Source: CAD feature listing. Evaluate the final solid. Frame: model axes, mm. A direction names the side the tool comes from. Round coordinates to 2 decimals unless told otherwise and drop trailing zeros. Loops run counter-clockwise (first coordinate to the right, second up) from the corner with the lowest first, then second, coordinate; pieces in that order, holes last. Notation, with made-up numbers: (51, 22) - (72, 22) arc R17 ccw to (72, 27) - close; hole circle Ø5 at (16.25, 52.25). An arc over 180 degrees is marked (long way). One line per question, with ' | ' between items. Start each with the question number.
1. Access query for faces 4 (the flat face through (20, 35, 1)), 5 (the flat face through (20, 59, 14)), 6 (the flat face through (20, 54, 19)). Directions: +Z, -Z, +X, -X, +Y, -Y. A direction counts if a zero-diameter tool reaches every point of the face in a straight line with its end or side. Return the directions, or none.
2. Cut plane B-B (x = 20). Return loops of the section in (y, z).
3. Mould query, pull axis Z, two halves, no side actions, for faces 1 (the flat face through (20, 5, -20)), 2 (the cylindrical face through (37.038, 56.535, 18.996)), 3 (the flat face through (20, 27, 6)). Classes: pulls with the +Z half, pulls with the -Z half, needs draft (parallel to the pull), parting line crosses it, or undercut.
4. Ray query, line 1 (X direction, y = 57, z = 17); line 2 (Z direction, x = 8, y = 6.95); line 3 (Z direction, x = 4, y = 55). Return the intervals inside material, ascending.
5. Cut plane C-C (z = -14). Return loops of the section in (x, y).
6. Cut plane D-D (y = 8). Return loops of the section in (x, z), then the cut area to 3 significant figures.
7. Cut plane A-A (z = -32). Return loops of the section in (x, y).
8. Pin query (flat end, axial travel): pin 1 (3.5 mm diameter, centred on x = 36, z = 17, fed in from +Y); pin 2 (17.5 mm diameter, centred on x = 21, z = 17, fed in from -Y); pin 3 (9 mm diameter, centred on x = 20, z = -32, fed in from +Y); pin 4 (7 mm diameter, centred on x = 4, z = 17, fed in from -Y). Return the tip coordinate at first contact, or that it passes through.
```python
from build123d import *

# Parameters (mm, degrees)
SKETCH1_W           = 52
SKETCH1_H           = 52
SKETCH1_W_2         = 42
SKETCH1_H_2         = 42
BOSS_EXTRUDE1_DEPTH = 5
SKETCH2_W           = 52
SKETCH2_H           = 52
BOSS_EXTRUDE2_DEPTH = 5
SKETCH3_W           = 52
SKETCH3_H           = 5
BOSS_EXTRUDE3_DEPTH = 44
SKETCH4_W           = 52
SKETCH4_H           = 26
BOSS_EXTRUDE4_DEPTH = 5
SKETCH5_R           = 2.25
CUT_EXTRUDE1_DEPTH  = 60
FILLET1_R           = 5
FILLET2_R           = 1
SKETCH7_R           = 4
CUT_EXTRUDE2_DEPTH  = 55
SKETCH8_W           = 52
SKETCH8_H           = 52
SKETCH8_W_2         = 42
SKETCH8_H_2         = 42
CUT_EXTRUDE3_DEPTH  = 5


with BuildPart() as part:
    # Sketch1 → Boss-Extrude1 (new body)
    with BuildSketch(Plane(origin=(0, 0, 0), x_dir=(1, 0, 0), z_dir=(0, 1, 0))):
        with Locations((20, 20)):
            Rectangle(SKETCH1_W, SKETCH1_H)
        with Locations((20, 20)):
            Rectangle(SKETCH1_W_2, SKETCH1_H_2, mode=Mode.SUBTRACT)
    extrude(amount=BOSS_EXTRUDE1_DEPTH)

    # Sketch2 → Boss-Extrude2 (add)
    with BuildSketch(Plane(origin=(0, 5, 0), x_dir=(1, 0, 0), z_dir=(0, 1, 0))):
        with Locations((20, 20)):
            Rectangle(SKETCH2_W, SKETCH2_H)
    extrude(amount=BOSS_EXTRUDE2_DEPTH)

    # Sketch3 → Boss-Extrude3 (add)
    with BuildSketch(Plane(origin=(0, 10, 0), x_dir=(1, 0, 0), z_dir=(0, 1, 0))):
        with Locations((20, -3.5)):
            Rectangle(SKETCH3_W, SKETCH3_H)
    extrude(amount=BOSS_EXTRUDE3_DEPTH)

    # Sketch4 → Boss-Extrude4 (add)
    with BuildSketch(Plane(origin=(0, 54, 0), x_dir=(1, 0, 0), z_dir=(0, 1, 0))):
        with Locations((20, -14)):
            Rectangle(SKETCH4_W, SKETCH4_H)
    extrude(amount=BOSS_EXTRUDE4_DEPTH)

    # Sketch5 → Cut-Extrude1 (cut, through all)
    with BuildSketch(Plane(origin=(0, 59, 0), x_dir=(1, 0, 0), z_dir=(0, 1, 0))):
        with Locations((36, -17)):
            Circle(SKETCH5_R)
        with Locations((4, -17)):
            Circle(SKETCH5_R)
    extrude(amount=-CUT_EXTRUDE1_DEPTH, mode=Mode.SUBTRACT)

    # Fillet1
    fillet1_edges = [part.edges().sort_by_distance(p)[0] for p in [
        (20, 54, 6),
    ]]
    fillet(fillet1_edges, radius=FILLET1_R)

    # Fillet2
    fillet2_edges = [part.edges().sort_by_distance(p)[0] for p in [
        (20, 10, 1),
    ]]
    fillet(fillet2_edges, radius=FILLET2_R)

    # Sketch7 → Cut-Extrude2 (cut, through all)
    with BuildSketch(Plane.XZ.offset(-5)):
        with Locations((20, -32)):
            Circle(SKETCH7_R)
        with Locations((32, -14)):
            Circle(SKETCH7_R)
        with Locations((8, -14)):
            Circle(SKETCH7_R)
    extrude(amount=-CUT_EXTRUDE2_DEPTH, mode=Mode.SUBTRACT)

    # Sketch8 → Cut-Extrude3 (cut)
    with BuildSketch(Plane.XZ):
        with Locations((20, -20)):
            Rectangle(SKETCH8_W, SKETCH8_H)
        with Locations((20, -20)):
            Rectangle(SKETCH8_W_2, SKETCH8_H_2, mode=Mode.SUBTRACT)
    extrude(amount=-CUT_EXTRUDE3_DEPTH, mode=Mode.SUBTRACT)


solid = part.part
```
Answers follow:
1) face 4: -Z, +X, -X, +Y | face 5: +Z, -Z, +X, -X, +Y | face 6: +Z, +X, -X, -Y
2) outline: (5, -46) - (10, -46) - (10, -36) - (5, -36) - close; (5, -28) - (10, -28) - (10, 0) arc R1 cw to (11, 1) - (59, 1) - (59, 27) - (54, 27) - (54, 11) arc R5 cw to (49, 6) - (5, 6) - close
3) face 1: needs draft | face 2: undercut | face 3: pulls with the +Z half
4) line 1: x = -6 to 1.75, 6.25 to 33.75, 38.25 to 46 | line 2: z = -46 to -18, -10 to 6 | line 3: z = 1 to 14.75, 19.25 to 27
5) outline: (-6, 5) - (4, 5) - (4, 10) - (-6, 10) - close; (12, 5) - (28, 5) - (28, 10) - (12, 10) - close; (36, 5) - (46, 5) - (46, 10) - (36, 10) - close
6) outline: (-6, -46) - (46, -46) - (46, 6) - (-6, 6) - close; hole circle Ø8 at (8, -14); hole circle Ø8 at (20, -32); hole circle Ø8 at (32, -14) | area: 2,550 mm2
7) outline: (-6, 5) - (16, 5) - (16, 10) - (-6, 10) - close; (24, 5) - (46, 5) - (46, 10) - (24, 10) - close
8) pin 1: passes through | pin 2: stops at y = 53.18 | pin 3: stops at y = 10 | pin 4: stops at y = 54
